from build123d import *

# Parameters (mm, degrees)
F1_DEPTH = 457.2
F2_W     = 5.08
F2_H     = 19.05
F3_DEPTH = 3.175


# Not quite as in the source:
# - a length typed as a fraction of an inch, garbled in the dataset ("3 / 203.2 mm" for 3/8 in), is restored


with BuildPart() as f1:
    # F0 (on Front) → F1 (new body, symmetric)
    with BuildSketch(Plane.XZ):
        Polygon((-76.2, 0), (0, 0), (42.8860933474, 0), (42.8860933474, 54.9768594564), (25.0777639449, 76.2), (0, 76.2), align=None)
    extrude(amount=F1_DEPTH, both=True)

    # F2 (on face) → F3 (join)
    with BuildSketch(Plane(origin=(-38.1, 0, 38.1), x_dir=(0, -1, 0), z_dir=(-0.7071067812, 0, 0.7071067812))):
        with BuildLine():
            Line((-391.6987875515, 28.4815367264), (-417.0987875515, 28.4815367264))
            ThreePointArc((-417.0987875515, 28.4815367264), (-431.8, -3.2684632736), (-417.0987875515, -35.0184632736))
            Line((-417.0987875515, -35.0184632736), (-391.6987875515, -35.0184632736))
            ThreePointArc((-391.6987875515, -35.0184632736), (-376.9975751031, -3.2684632736), (-391.6987875515, 28.4815367264))
        make_face()
        with BuildLine():
            Line((-400.5195509719, -30.7538155466), (-409.9965240192, -30.7538155466))
            Line((-409.9965240192, -30.7538155466), (-409.9965240192, -25.4346902415))
            ThreePointArc((-409.9965240192, -25.4346902415), (-405.2253041336, -20.6960921992), (-400.5195509719, -25.4997093556))
            Line((-400.5195509719, -25.4997093556), (-400.5195509719, -30.7538155466))
        make_face(mode=Mode.SUBTRACT)
        with Locations((-412.5365240192, 2.0394300796)):
            Rectangle(F2_W, F2_H, mode=Mode.SUBTRACT)
        with Locations((-397.9795509719, 2.4147130909)):
            Rectangle(F2_W, F2_H, mode=Mode.SUBTRACT)
        with BuildLine():
            Line((-264.41702, 28.96613), (-289.81702, 28.96613))
            ThreePointArc((-289.81702, 28.96613), (-304.5182324485, -2.78387), (-289.81702, -34.53387))
            Line((-289.81702, -34.53387), (-264.41702, -34.53387))
            ThreePointArc((-264.41702, -34.53387), (-249.7158075515, -2.78387), (-264.41702, 28.96613))
        make_face()
        with BuildLine():
            Line((-272.8882718836, -29.7792267651), (-282.365244931, -29.7792267651))
            Line((-282.365244931, -29.7792267651), (-282.365244931, -24.46010146))
            ThreePointArc((-282.365244931, -24.46010146), (-277.5940250453, -19.7215034177), (-272.8882718836, -24.5251205741))
            Line((-272.8882718836, -24.5251205741), (-272.8882718836, -29.7792267651))
        make_face(mode=Mode.SUBTRACT)
        with Locations((-284.905244931, 3.0140188611)):
            Rectangle(F2_W, F2_H, mode=Mode.SUBTRACT)
        with Locations((-270.3482718836, 3.3893018724)):
            Rectangle(F2_W, F2_H, mode=Mode.SUBTRACT)
        with BuildLine():
            Line((-137.1352524485, 29.4507232736), (-162.5352524485, 29.4507232736))
            ThreePointArc((-162.5352524485, 29.4507232736), (-177.2364648969, -2.2992767264), (-162.5352524485, -34.0492767264))
            Line((-162.5352524485, -34.0492767264), (-137.1352524485, -34.0492767264))
            ThreePointArc((-137.1352524485, -34.0492767264), (-122.43404, -2.2992767264), (-137.1352524485, 29.4507232736))
        make_face()
        with BuildLine():
            Line((-145.2569927954, -28.8046379836), (-154.7339658427, -28.8046379836))
            Line((-154.7339658427, -28.8046379836), (-154.7339658427, -23.4855126785))
            ThreePointArc((-154.7339658427, -23.4855126785), (-149.962745957, -18.7469146362), (-145.2569927954, -23.5505317926))
            Line((-145.2569927954, -23.5505317926), (-145.2569927954, -28.8046379836))
        make_face(mode=Mode.SUBTRACT)
        with Locations((-157.2739658427, 3.9886076427)):
            Rectangle(F2_W, F2_H, mode=Mode.SUBTRACT)
        with Locations((-142.7169927954, 4.3638906539)):
            Rectangle(F2_W, F2_H, mode=Mode.SUBTRACT)
        with BuildLine():
            Line((-9.8534848969, 29.9353165472), (-35.2534848969, 29.9353165472))
            ThreePointArc((-35.2534848969, 29.9353165472), (-49.9546973454, -1.8146834528), (-35.2534848969, -33.5646834528))
            Line((-35.2534848969, -33.5646834528), (-9.8534848969, -33.5646834528))
            ThreePointArc((-9.8534848969, -33.5646834528), (4.8477275515, -1.8146834528), (-9.8534848969, 29.9353165472))
        make_face()
        with BuildLine():
            Line((-17.6257137071, -27.8300492021), (-27.1026867544, -27.8300492021))
            Line((-27.1026867544, -27.8300492021), (-27.1026867544, -22.5109238969))
            ThreePointArc((-27.1026867544, -22.5109238969), (-22.3314668688, -17.7723258546), (-17.6257137071, -22.575943011))
            Line((-17.6257137071, -22.575943011), (-17.6257137071, -27.8300492021))
        make_face(mode=Mode.SUBTRACT)
        with Locations((-29.6426867544, 4.9631964242)):
            Rectangle(F2_W, F2_H, mode=Mode.SUBTRACT)
        with Locations((-15.0857137071, 5.3384794355)):
            Rectangle(F2_W, F2_H, mode=Mode.SUBTRACT)
        with BuildLine():
            Line((117.4282826546, 30.4199098208), (92.0282826546, 30.4199098208))
            ThreePointArc((92.0282826546, 30.4199098208), (77.3270702061, -1.3300901792), (92.0282826546, -33.0800901792))
            Line((92.0282826546, -33.0800901792), (117.4282826546, -33.0800901792))
            ThreePointArc((117.4282826546, -33.0800901792), (132.1294951031, -1.3300901792), (117.4282826546, 30.4199098208))
        make_face()
        with BuildLine():
            Line((110.0055653812, -26.8554604205), (100.5285923338, -26.8554604205))
            Line((100.5285923338, -26.8554604205), (100.5285923338, -21.5363351154))
            ThreePointArc((100.5285923338, -21.5363351154), (105.2998122195, -16.7977370731), (110.0055653812, -21.6013542295))
            Line((110.0055653812, -21.6013542295), (110.0055653812, -26.8554604205))
        make_face(mode=Mode.SUBTRACT)
        with Locations((97.9885923338, 5.9377852057)):
            Rectangle(F2_W, F2_H, mode=Mode.SUBTRACT)
        with Locations((112.5455653812, 6.313068217)):
            Rectangle(F2_W, F2_H, mode=Mode.SUBTRACT)
        with BuildLine():
            Line((244.7100502061, 30.9045030943), (219.3100502061, 30.9045030943))
            ThreePointArc((219.3100502061, 30.9045030943), (204.6088377576, -0.8454969057), (219.3100502061, -32.5954969057))
            Line((219.3100502061, -32.5954969057), (244.7100502061, -32.5954969057))
            ThreePointArc((244.7100502061, -32.5954969057), (259.4112626546, -0.8454969057), (244.7100502061, 30.9045030943))
        make_face()
        with BuildLine():
            Line((237.6368444694, -25.880871639), (228.1598714221, -25.880871639))
            Line((228.1598714221, -25.880871639), (228.1598714221, -20.5617463339))
            ThreePointArc((228.1598714221, -20.5617463339), (232.9310913078, -15.8231482916), (237.6368444694, -20.626765448))
            Line((237.6368444694, -20.626765448), (237.6368444694, -25.880871639))
        make_face(mode=Mode.SUBTRACT)
        with Locations((225.6198714221, 6.9123739872)):
            Rectangle(F2_W, F2_H, mode=Mode.SUBTRACT)
        with Locations((240.1768444694, 7.2876569985)):
            Rectangle(F2_W, F2_H, mode=Mode.SUBTRACT)
        with BuildLine():
            Line((371.9918177576, 31.3890963679), (346.5918177576, 31.3890963679))
            ThreePointArc((346.5918177576, 31.3890963679), (331.8906053092, -0.3609036321), (346.5918177576, -32.1109036321))
            Line((346.5918177576, -32.1109036321), (371.9918177576, -32.1109036321))
            ThreePointArc((371.9918177576, -32.1109036321), (386.6930302061, -0.3609036321), (371.9918177576, 31.3890963679))
        make_face()
        with BuildLine():
            Line((365.2681235577, -24.9062828575), (355.7911505104, -24.9062828575))
            Line((355.7911505104, -24.9062828575), (355.7911505104, -19.5871575524))
            ThreePointArc((355.7911505104, -19.5871575524), (360.562370396, -14.8485595101), (365.2681235577, -19.6521766665))
            Line((365.2681235577, -19.6521766665), (365.2681235577, -24.9062828575))
        make_face(mode=Mode.SUBTRACT)
        with Locations((353.2511505104, 7.8869627688)):
            Rectangle(F2_W, F2_H, mode=Mode.SUBTRACT)
        with Locations((367.8081235577, 8.26224578)):
            Rectangle(F2_W, F2_H, mode=Mode.SUBTRACT)
    extrude(amount=F3_DEPTH)


solid = f1.part
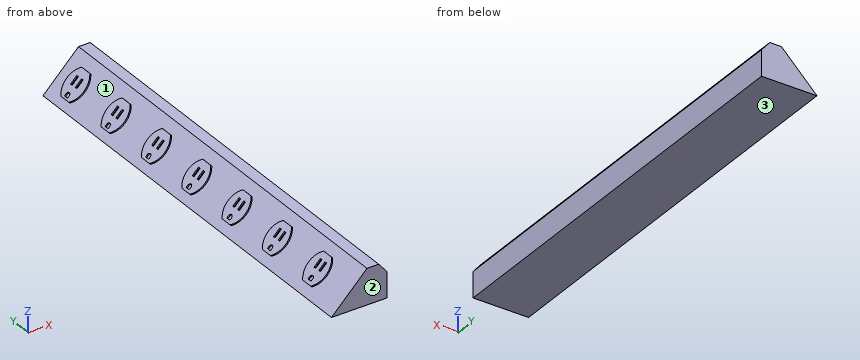
Read the model definition and answer for the solid it produces. Units are mm, in the model's axes. Face numbers are marked on the shaded views. Coordinates: 2 decimals unless noted, no trailing zeros. Order: outer loops, then holes, each group sorted by start corner. A loop starts at its lowest first (then second) coordinate and runs counter-clockwise, first axis right, second up. Notation, with made-up numbers: M 49,-35.5 L 53,-35.5 A21 cw 53,-1.5 Z; hole C -3,-28.75 d8. An arc over 180 degrees is marked long. Put each result on its own line as item: value. Start each with the question number.
Item 1: Section A-A, the plane y = 359.5 is taken. Determine the outline of the cut face in (x, z), plus the area to 3 significant figures.
Item 2: Consider probe 1 along X at (y, z) = (260.5, 15); probe 2 along X at (y, z) = (388.5, 50.5); probe 3 along Z at (x, y) = (-58.5, 305.5). Determine where each line is inside the solid, lowest interval first. Write a range as [from, to].
Item 3: Given pin 1 Ø4.5 at (x, z) = (-38, 43.5) entering from -Y; pin 2 Ø5 at (x, z) = (-58, 22) entering from +Y; pin 3 Ø1.5 at (x, y) = (-37.5, -158.5) entering from +Z, each flat-ended and moving along its own axis, determine where each tip first touches the part or whether it passes through.
Item 4: The mould has two halves that part along Y. Classify the marked faces 1, 2 and 3: +Y half, -Y half, draft (parallel to the pull), parting line (faces both ways), or undercut.
Computed:
1. outline: M -76.2,0 L 42.89,0 L 42.89,54.98 L 25.08,76.2 L 0,76.2 Z
1. area: 5,980 mm2
2. probe 1: x = [-61.2, 42.89]
2. probe 2: x = [-30.19, 42.89]
2. probe 3: z = [0, 17.7]
3. pin 1: stops at y = -386.64
3. pin 2: stops at y = 426.85
3. pin 3: stops at z = 39.45
4. face 1: undercut
4. face 2: -Y half
4. face 3: draft
